```python
from build123d import *

# Parameters (mm, degrees)
CYLINDER004_R     = 1
CYLINDER004_DEPTH = 10
ARRAY002_X_COUNT  = 2
ARRAY002_X_PITCH  = 65.5
ARRAY002_Y_COUNT  = 2
ARRAY002_Y_PITCH  = 45.5
BOX005_W          = 70
BOX005_H          = 50
BOX005_DEPTH      = 1.5


with BuildPart() as pcb_hole_array:
    # Cylinder004 → Cylinder004 (new body)
    with BuildSketch(Plane.XY):
        Circle(CYLINDER004_R)
    extrude(amount=CYLINDER004_DEPTH)

    # Array002 X: pcb hole array ×2


with BuildPart() as pcb_hole_array_1:
    add(pcb_hole_array.part)
    with Locations(*[(i * ARRAY002_X_PITCH, 0, 0) for i in range(1, ARRAY002_X_COUNT)]):
        add(pcb_hole_array.part)

    # Array002 Y: pcb hole array ×2


with BuildPart() as pcb_hole_array_2:
    add(pcb_hole_array_1.part)
    with Locations(*[(0, i * ARRAY002_Y_PITCH, 0) for i in range(1, ARRAY002_Y_COUNT)]):
        add(pcb_hole_array_1.part)


with BuildPart() as pcb_hole_array_3:
    # Array002 placement: moved
    add(pcb_hole_array_2.part.moved(Location((2.25, 2.25, 0))))


with BuildPart() as pcb_7x5_mockup_cut:
    # Box005 → Box005 (new body)
    with BuildSketch(Plane.XY):
        with Locations((35, 25)):
            Rectangle(BOX005_W, BOX005_H)
    extrude(amount=BOX005_DEPTH)

    # Cut002: cut pcb hole array
    add(pcb_hole_array_3.part, mode=Mode.SUBTRACT)


with BuildPart() as pcb_7x5_mockup_cut_1:
    # Cut002 placement: moved
    add(pcb_7x5_mockup_cut.part.moved(Location((7, 7, 5))))


solid = pcb_7x5_mockup_cut_1.part
```
Geometry check sheet. Reference: the model listing, model coordinates, mm. Round coordinates to 2 decimals unless told otherwise and drop trailing zeros. Loops run counter-clockwise (first coordinate to the right, second up) from the corner with the lowest first, then second, coordinate; pieces in that order, holes last. Notation, with made-up numbers: (-25, 52) -> (-7, 52) arc R13 cw to (-7, 75) -> close; hole circle Ø10 at (-39.75, -5.5). An arc over 180 degrees is marked (long way). Use a Markdown table: item, result.
(1) Scan lines: probe 1 along Y at (x, z) = (74.75, 6.2); probe 2 along X at (y, z) = (9.25, 6.1); probe 3 along X at (y, z) = (10, 6). Record each from-to range of solid material in increasing order.
Calculated:
| item | result |
|---|---|
| probe 1 | 7 to 8.25, 10.25 to 53.75, 55.75 to 57 |
| probe 2 | 7 to 8.25, 10.25 to 73.75, 75.75 to 77 |
| probe 3 | 7 to 8.59, 9.91 to 74.09, 75.41 to 77 |
(2) Sectioned sample at B-B (y = 54.75). Enter the section's corners in (x, z), then the cut area to 3 significant figures.
Calculated:
| item | result |
|---|---|
| outline | (7, 5) -> (8.25, 5) -> (8.25, 6.5) -> (7, 6.5) -> close; (10.25, 5) -> (73.75, 5) -> (73.75, 6.5) -> (10.25, 6.5) -> close; (75.75, 5) -> (77, 5) -> (77, 6.5) -> (75.75, 6.5) -> close |
| area | 99.0 mm² |
(3) Sectioned sample at A-A (x = 9.25). Enter the section's corners in (y, z).
Calculated:
| item | result |
|---|---|
| outline | (7, 5) -> (8.25, 5) -> (8.25, 6.5) -> (7, 6.5) -> close; (10.25, 5) -> (53.75, 5) -> (53.75, 6.5) -> (10.25, 6.5) -> close; (55.75, 5) -> (57, 5) -> (57, 6.5) -> (55.75, 6.5) -> close |
(4) Mould release check, pull along X, two halves, no side actions. Record for faces 1 (the flat face through (42, 7, 6)), 2 (the cylindrical face through (9.12, 55.74, 5.74)), 3 (the flat face through (7, 32, 6)): released by +X, released by -X, zero draft, split by the parting line, or undercut.
Calculated:
| item | result |
|---|---|
| face 1 | zero draft |
| face 2 | undercut |
| face 3 | released by -X |
